The figure shows three views and two pictorial views of one solid part (mm, origin at its lowest corner). Answer the questions. A direction names the side the tool comes from. Give positions to 0.01 mm unless a question says otherwise; leave off trailing zeros. Order: outer loops, then holes, each group sorted by start corner. A loop starts at its lowest first (then second) coordinate and runs counter-clockwise, first axis right, second up. Notation, with made-up numbers: M 59,63.5 L 63,63.5 A6 ccw 63,73.5 Z; hole C -20.5,38.25 d6. An arc over 180 degrees is marked long. Answer as a JSON object with one key per item and string values. Group by question number.
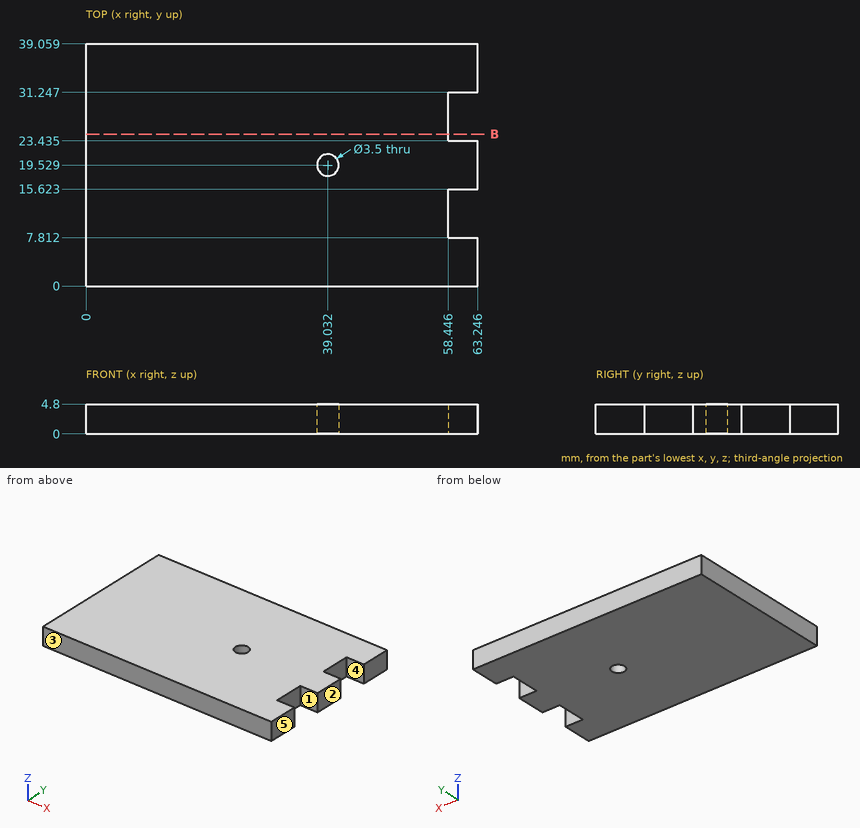
Item 1: A flat-ended cylindrical pin translates along its axis: P1, Ø1.4, axis at y = 11.5, z = 1.5, coming from the +X side. Find the tip coordinate at first contact, or state that the pin passes through.
Item 2: Consider probe 1 along Y at (x, z) = (58.5, 1.45) (1 decimal); probe 2 along X at (y, z) = (24.5, 1.9). Determine where each line is inside the solid, lowest interval first. Write a range as from..to.
Item 3: Determine the mould class of the marked faces 3, 4 and 5 for opening direction Y: released by +Y, released by -Y, zero draft, split by the parting line, or undercut.
Item 4: A tool of negligible diameter and unlimited length cuts with its end or side. For the marked faces 1 and 2, from which of +Z, -Z, +X, -X, +Y, -Y can it reach the whole face along a straight path? Write none if from no direction.
Item 5: Section B-B (y = 24.5) is taken. Determine the outline of the cut face in (x, z).
Values found:
{
 "1": {"P1": "stops at x = 58.45"},
 "2": {"probe 1": "y = 0..7.8, 15.6..23.4, 31.2..39.1", "probe 2": "x = 0..58.45"},
 "3": {"face 3": "released by -Y", "face 4": "undercut", "face 5": "zero draft"},
 "4": {"face 1": "+Z, -Z, +X", "face 2": "+Z, -Z, +X, +Y, -Y"},
 "5": {"outline": "M 0,0 L 58.45,0 L 58.45,4.8 L 0,4.8 Z"}
}
